For this review, take the finished solid that the model builds, in its own axes (mm). A direction names the side the tool comes from. Round coordinates to 2 decimals unless told otherwise and drop trailing zeros. Order: outer loops, then holes, each group sorted by start corner. A loop starts at its lowest first (then second) coordinate and runs counter-clockwise, first axis right, second up. Notation, with made-up numbers: M 65,33.25 L 124,33.25 A18 ccw 124,43.25 Z; hole C -9,68.25 d6. An arc over 180 degrees is marked long. Answer as a JSON object with one key per item and string values.
from build123d import *

# Parameters (mm, degrees)
SKETCH3_W           = 118.5
SKETCH3_H           = 144
BOSS_EXTRUDE1_DEPTH = 30
SKETCH4_R           = 11
CUT_EXTRUDE1_DEPTH  = 2
SKETCH5_R           = 4
CUT_EXTRUDE2_DEPTH  = 30
SKETCH7_W           = 41
SKETCH7_H           = 177.768192582
CUT_EXTRUDE4_DEPTH  = 20
SKETCH8_W           = 86.017782004
SKETCH8_H           = 50
CUT_EXTRUDE5_DEPTH  = 20
SKETCH9_R           = 7.5
CUT_EXTRUDE6_DEPTH  = 30
SKETCH10_W          = 32
SKETCH10_H          = 32
CUT_EXTRUDE7_DEPTH  = 15
SKETCH14_R          = 2
CUT_EXTRUDE10_DEPTH = 15
SKETCH15_R          = 2
CUT_EXTRUDE11_DEPTH = 34
SKETCH16_R          = 4
CUT_EXTRUDE12_DEPTH = 26
SKETCH17_W          = 32
SKETCH17_H          = 32
BOSS_EXTRUDE2_DEPTH = 15
SKETCH18_W          = 10
SKETCH18_H          = 30
BOSS_EXTRUDE3_DEPTH = 144
SKETCH19_W          = 22
SKETCH19_H          = 30
CUT_EXTRUDE13_DEPTH = 144
SKETCH20_R          = 2
CUT_EXTRUDE14_DEPTH = 10
SKETCH21_R          = 7.75
CUT_EXTRUDE15_DEPTH = 15
SKETCH22_R          = 4
CUT_EXTRUDE16_DEPTH = 4
SKETCH23_R          = 4
CUT_EXTRUDE17_DEPTH = 4
BOSS_EXTRUDE4_START = -10
SKETCH24_R          = 2
BOSS_EXTRUDE4_DEPTH = 10
SKETCH25_R          = 5
CUT_EXTRUDE18_DEPTH = 10
SKETCH26_R          = 1.5
CUT_EXTRUDE19_DEPTH = 15
SKETCH27_R          = 11.25
CUT_EXTRUDE20_DEPTH = 2
SKETCH28_W          = 50
SKETCH28_H          = 50
SKETCH28_R          = 18.25
BOSS_EXTRUDE5_DEPTH = 23
SKETCH29_R          = 1.5
CUT_EXTRUDE21_DEPTH = 10
FILLET1_R           = 2


with BuildPart() as part:
    # Sketch3 → Boss-Extrude1 (new body)
    with BuildSketch(Plane.XY):
        Rectangle(SKETCH3_W, SKETCH3_H)
    extrude(amount=-BOSS_EXTRUDE1_DEPTH)

    # Sketch4 → Cut-Extrude1 (cut)
    with BuildSketch(Plane.XY):
        with Locations((34.25, 0)):
            Circle(SKETCH4_R)
    extrude(amount=-CUT_EXTRUDE1_DEPTH, mode=Mode.SUBTRACT)

    # Sketch5 → Cut-Extrude2 (cut)
    with BuildSketch(Plane.XY.offset(-2)):
        with Locations((34.25, 0)):
            Circle(SKETCH5_R)
    extrude(amount=-CUT_EXTRUDE2_DEPTH, mode=Mode.SUBTRACT)

    # Sketch7 → Cut-Extrude4 (cut)
    with BuildSketch(Plane(origin=(0, 0, -30), x_dir=(-1, 0, 0), z_dir=(0, 0, -1))):
        with Locations((6.75, 0)):
            Rectangle(SKETCH7_W, SKETCH7_H)
    extrude(amount=-CUT_EXTRUDE4_DEPTH, mode=Mode.SUBTRACT)

    # Sketch8 → Cut-Extrude5 (cut)
    with BuildSketch(Plane(origin=(0, 0, -30), x_dir=(-1, 0, 0), z_dir=(0, 0, -1))):
        with Locations((-34.25, 0)):
            Rectangle(SKETCH8_W, SKETCH8_H)
    extrude(amount=-CUT_EXTRUDE5_DEPTH, mode=Mode.SUBTRACT)

    # Sketch9 → Cut-Extrude6 (cut)
    with BuildSketch(Plane.XY):
        with Locations((-43.25, 0)):
            Circle(SKETCH9_R)
        with Locations((43.25, -56)):
            Circle(SKETCH9_R)
        with Locations((43.25, 56)):
            Circle(SKETCH9_R)
    extrude(amount=-CUT_EXTRUDE6_DEPTH, mode=Mode.SUBTRACT)

    # Sketch10 → Cut-Extrude7 (cut)
    with BuildSketch(Plane.XY):
        with Locations((-43.25, 0)):
            Rectangle(SKETCH10_W, SKETCH10_H)
        with Locations((43.25, 56)):
            Rectangle(SKETCH10_W, SKETCH10_H)
        with Locations((43.25, -56)):
            Rectangle(SKETCH10_W, SKETCH10_H)
    extrude(amount=-CUT_EXTRUDE7_DEPTH, mode=Mode.SUBTRACT)

    # Sketch14 → Cut-Extrude10 (cut)
    with BuildSketch(Plane(origin=(0, 0, -10), x_dir=(-1, 0, 0), z_dir=(0, 0, -1))):
        with Locations((16.75, 0)):
            Circle(SKETCH14_R)
        with Locations((-3.25, 0)):
            Circle(SKETCH14_R)
        with Locations((16.75, 57)):
            Circle(SKETCH14_R)
        with Locations((-3.25, 57)):
            Circle(SKETCH14_R)
        with Locations((16.75, -57)):
            Circle(SKETCH14_R)
        with Locations((-3.25, -57)):
            Circle(SKETCH14_R)
    extrude(amount=-CUT_EXTRUDE10_DEPTH, mode=Mode.SUBTRACT)

    # Sketch15 → Cut-Extrude11 (cut)
    with BuildSketch(Plane.ZY.offset(59.25)):
        with Locations((-20, 44)):
            Circle(SKETCH15_R)
        with Locations((-20, -44)):
            Circle(SKETCH15_R)
    extrude(amount=-CUT_EXTRUDE11_DEPTH, mode=Mode.SUBTRACT)

    # Sketch16 → Cut-Extrude12 (cut)
    with BuildSketch(Plane.ZY.offset(59.25)):
        with Locations((-20, 44)):
            Circle(SKETCH16_R)
        with Locations((-20, -44)):
            Circle(SKETCH16_R)
    extrude(amount=-CUT_EXTRUDE12_DEPTH, mode=Mode.SUBTRACT)

    # Sketch17 → Boss-Extrude2 (add)
    with BuildSketch(Plane.XY.offset(-15)):
        with Locations((-43.25, 0)):
            Rectangle(SKETCH17_W, SKETCH17_H)
    extrude(amount=BOSS_EXTRUDE2_DEPTH)

    # Sketch18 → Boss-Extrude3 (add)
    with BuildSketch(Plane(origin=(0, 72, 0), x_dir=(1, 0, 0), z_dir=(0, 1, 0))):
        with Locations((-32.25, 15)):
            Rectangle(SKETCH18_W, SKETCH18_H)
    extrude(amount=-BOSS_EXTRUDE3_DEPTH)

    # Sketch19 → Cut-Extrude13 (cut)
    with BuildSketch(Plane(origin=(0, 72, 0), x_dir=(1, 0, 0), z_dir=(0, 1, 0))):
        with Locations((-48.25, 15)):
            Rectangle(SKETCH19_W, SKETCH19_H)
    extrude(amount=-CUT_EXTRUDE13_DEPTH, mode=Mode.SUBTRACT)

    # Sketch20 → Cut-Extrude14 (cut)
    with BuildSketch(Plane(origin=(-27.25, 0, 0), x_dir=(0, 0, -1), z_dir=(1, 0, 0))):
        with Locations((20, -50)):
            Circle(SKETCH20_R)
        with Locations((20, 0)):
            Circle(SKETCH20_R)
        with Locations((20, 50)):
            Circle(SKETCH20_R)
    extrude(amount=-CUT_EXTRUDE14_DEPTH, mode=Mode.SUBTRACT)

    # Sketch21 → Cut-Extrude15 (cut)
    with BuildSketch(Plane.XY.offset(-15)):
        with Locations((43.25, -56)):
            Circle(SKETCH21_R)
        with Locations((43.25, 56)):
            Circle(SKETCH21_R)
    extrude(amount=-CUT_EXTRUDE15_DEPTH, mode=Mode.SUBTRACT)

    # Sketch22 → Cut-Extrude16 (cut)
    with BuildSketch(Plane.ZY.offset(37.25)):
        with Locations((-20, 50)):
            Circle(SKETCH22_R)
        with Locations((-20, 0)):
            Circle(SKETCH22_R)
        with Locations((-20, -50)):
            Circle(SKETCH22_R)
    extrude(amount=-CUT_EXTRUDE16_DEPTH, mode=Mode.SUBTRACT)

    # Sketch23 → Cut-Extrude17 (cut)
    with BuildSketch(Plane.XY):
        with Locations((-16.75, 57)):
            Circle(SKETCH23_R)
        with Locations((3.25, 57)):
            Circle(SKETCH23_R)
        with Locations((-16.75, -57)):
            Circle(SKETCH23_R)
        with Locations((3.25, -57)):
            Circle(SKETCH23_R)
    extrude(amount=-CUT_EXTRUDE17_DEPTH, mode=Mode.SUBTRACT)

    # Sketch24 → Boss-Extrude4 (add)
    with BuildSketch(Plane.XY.offset(BOSS_EXTRUDE4_START)):
        with Locations((-16.75, 0)):
            Circle(SKETCH24_R)
        with Locations((3.25, 0)):
            Circle(SKETCH24_R)
    extrude(amount=BOSS_EXTRUDE4_DEPTH)

    # Sketch25 → Cut-Extrude18 (cut)
    with BuildSketch(Plane.XY.offset(-2)):
        with Locations((34.25, 0)):
            Circle(SKETCH25_R)
    extrude(amount=-CUT_EXTRUDE18_DEPTH, mode=Mode.SUBTRACT)

    # Sketch26 → Cut-Extrude19 (cut)
    with BuildSketch(Plane.XY.offset(-15)):
        with Locations((34.764718626, -64.485281374)):
            Circle(SKETCH26_R)
        with Locations((34.764718626, -47.514718626)):
            Circle(SKETCH26_R)
        with Locations((51.735281374, -47.514718626)):
            Circle(SKETCH26_R)
        with Locations((51.735281374, -64.485281374)):
            Circle(SKETCH26_R)
        with Locations((34.764718626, 47.514718626)):
            Circle(SKETCH26_R)
        with Locations((51.735281374, 47.514718626)):
            Circle(SKETCH26_R)
        with Locations((51.735281374, 64.485281374)):
            Circle(SKETCH26_R)
        with Locations((34.764718626, 64.485281374)):
            Circle(SKETCH26_R)
    extrude(amount=-CUT_EXTRUDE19_DEPTH, mode=Mode.SUBTRACT)

    # Sketch27 → Cut-Extrude20 (cut)
    with BuildSketch(Plane.XY):
        with Locations((34.25, 0)):
            Circle(SKETCH27_R)
    extrude(amount=-CUT_EXTRUDE20_DEPTH, mode=Mode.SUBTRACT)

    # Sketch28 → Boss-Extrude5 (add)
    with BuildSketch(Plane.XY):
        with Locations((34.25, 0)):
            Rectangle(SKETCH28_W, SKETCH28_H)
        with Locations((34.25, 0)):
            Circle(SKETCH28_R, mode=Mode.SUBTRACT)
    extrude(amount=BOSS_EXTRUDE5_DEPTH)

    # Sketch29 → Cut-Extrude21 (cut)
    with BuildSketch(Plane(origin=(0, 0, -10), x_dir=(-1, 0, 0), z_dir=(0, 0, -1))):
        with Locations((-23.643398282, 10.606601718)):
            Circle(SKETCH29_R)
        with Locations((-23.643398282, -10.606601718)):
            Circle(SKETCH29_R)
        with Locations((-44.856601718, 10.606601718)):
            Circle(SKETCH29_R)
        with Locations((-44.856601718, -10.606601718)):
            Circle(SKETCH29_R)
    extrude(amount=-CUT_EXTRUDE21_DEPTH, mode=Mode.SUBTRACT)

    # Fillet1
    fillet1_edges = [part.edges().sort_by_distance(p)[0] for p in [
        (-37.25, 72, -15),
        (-37.25, -72, -15),
        (-37.25, 0, -30),
        (-37.25, 0, 0),
        (43.25, -72, -15),
        (36.5, -72, -30),
        (36.5, -25, -30),
        (36.5, 25, -30),
        (36.5, 72, -30),
        (-5, 72, 0),
        (27.25, 56, 0),
        (43.25, 40, 0),
        (59.25, 25, 11.5),
        (9.25, 25, 11.5),
        (9.25, -25, 11.5),
        (34.25, 25, 23),
        (9.25, 0, 23),
        (34.25, -25, 23),
        (59.25, 0, 23),
        (59.25, -25, 11.5),
        (43.25, -40, 0),
        (27.25, -56, 0),
        (27.25, -72, -7.5),
        (59.25, -40, -7.5),
        (27.25, 72, -7.5),
        (59.25, 40, -7.5),
        (59.25, 72, -22.5),
        (59.25, 48.5, -30),
        (59.25, 25, -20),
        (59.25, -48.5, -30),
        (59.25, -25, -20),
        (59.25, -72, -22.5),
        (-5, -72, 0),
        (59.25, -56, -15),
        (59.25, 56, -15),
        (59.25, 32.5, 0),
        (59.25, -32.5, 0),
        (43.25, 72, -15),
    ]]
    fillet(fillet1_edges, radius=FILLET1_R)


solid = part.part
1) Add section B-B on y = 0. State how many separate pieces and enclosed holes the cut face has, and give its area (3 significant figures).
Geometry check:
{"separate pieces": "3", "enclosed holes": "0", "area": "1,290 mm²"}
2) Add section A-A on x = 3.25. State the section outline as (y, z) points.
Geometry check:
{"outline": "M -72,-10 L -59,-10 L -59,-4 L -61,-4 L -61,0 L -70,0 A2 ccw -72,-2 Z; M -55,-10 L 55,-10 L 55,-4 L 53,-4 L 53,0 L -53,0 L -53,-4 L -55,-4 Z; M 59,-10 L 72,-10 L 72,-2 A2 ccw 70,0 L 61,0 L 61,-4 L 59,-4 Z"}
3) Add section C-C on x = -30.5. State the section outline as (y, z) points, and give its area (3 significant figures).
Geometry check:
{"outline": "M -72,-30 L 72,-30 L 72,-2 A2 ccw 70,0 L -70,0 A2 ccw -72,-2 Z; hole C -50,-20 d4; hole C 0,-20 d4; hole C 50,-20 d4", "area": "4,280 mm²"}
4) Add section D-D on z = 5. State the section outline as (x, y) points, and give its area (3 significant figures).
Geometry check:
{"outline": "M 9.25,-23 A2 ccw 11.25,-25 L 57.25,-25 A2 ccw 59.25,-23 L 59.25,23 A2 ccw 57.25,25 L 11.25,25 A2 ccw 9.25,23 Z; hole C 34.25,0 d36.5", "area": "1,450 mm²"}
5) Insertion check: P1, Ø6.5, axis at y = -48, z = -18.5, coming from the -X side; P2, Ø3.5, axis at x = 34.76, y = -64.49, coming from the +Z side; P3, Ø5, axis at x = 3.25, y = -57, coming from the +Z side; P4, Ø6, axis at x = 31, z = -5.5, coming from the -Y side. Each pin has a flat end and moves straight along its axis. Give the tip position at first contact, or say it passes through.
Geometry check:
{"P1": "stops at x = -37.25", "P2": "stops at z = -15", "P3": "stops at z = -4", "P4": "stops at y = -40"}
6) Machinability: for faces 1 (the flat face through (-19, 56, -4)), 2 (the flat face through (36, -25, -19)), 3 (the flat face through (34, 25, 10)), 4 (the cylindrical face through (-35.3, -52.4, -23.2)), 5 (the cylindrical face through (50.545, -65.398, -22.395)), which of the approach directions +Z, -Z, +X, -X, +Y, -Y give a long, thin tool a straight path to every point of the face, cutting with its end or side? Answer none if there is none.
Geometry check:
{"face 1": "+Z", "face 2": "-Z, +X", "face 3": "+Z, +X, -X, +Y", "face 4": "-X", "face 5": "+Z, -Z"}
7) For L1, parallel to Y at x = -16.75, z = -5.15; L2, parallel to Y at x = -30.55, z = -20; L3, parallel to Y at x = -34, z = -20, list the stretches that pass through material, from the lowest coordinate up.
Geometry check:
{"L1": "y = -72 to -59, -55 to 55, 59 to 72", "L2": "y = -72 to -52, -48 to -2, 2 to 48, 52 to 72", "L3": "y = -72 to -54, -46 to -4, 4 to 46, 54 to 72"}
8) Mouldability with a two-part tool opening along X and no side actions: class faces 6 (the cylindrical face through (50.545, 63.573, -22.395)), 7 (the flat face through (35, 55, -15)), 8 (the flat face through (-37.25, 1, -15)) as +X half, -X half, draft (parallel to the pull), parting line (faces both ways), or undercut.
Geometry check:
{"face 6": "undercut", "face 7": "draft", "face 8": "-X half"}
